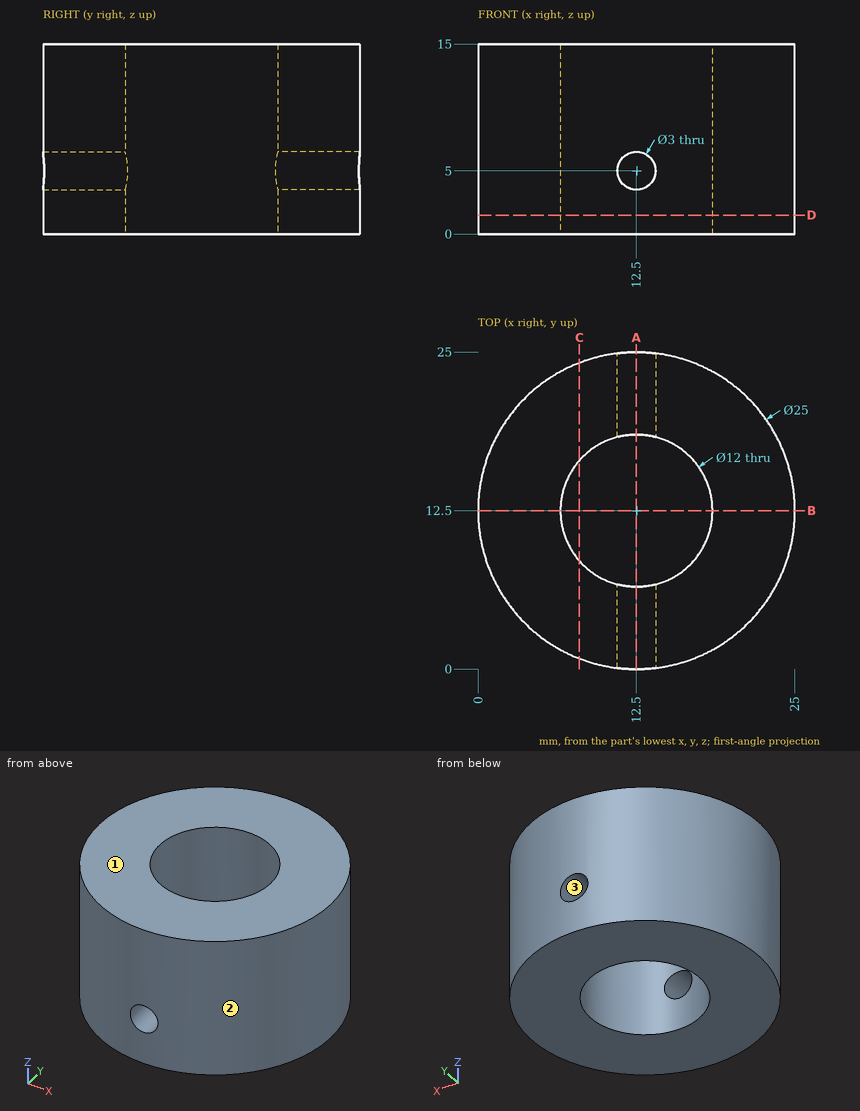
Source: three-view drawing plus pictorial views. Frame: mm from the lowest corner of the part. Round coordinates to 2 decimals unless told otherwise and drop trailing zeros. Loops run counter-clockwise (first coordinate to the right, second up) from the corner with the lowest first, then second, coordinate; pieces in that order, holes last.
1. Section query C-C on x = 8. Output: boundary loops of the cut face in (y, z), and give its area (3 significant figures).
2. Ray query, L1, parallel to Y at x = 12.5, z = 10.5; L2, parallel to Z at x = 12.5, y = 23; L3, parallel to Y at x = 14.25, z = 9.75. Return the intervals inside material, ascending.
3. Section query A-A on x = 12.5. Output: boundary loops of the cut face in (y, z), and give its area (3 significant figures).
4. Section query D-D on z = 1.5. Output: boundary loops of the cut face in (x, y).
5. Contact query for flat-ended pins moving along their axis: pin 1 (3 mm diameter, centred on x = 7.5, z = 13.5, fed in from +Y); pin 2 (14 mm diameter, centred on x = 12.5, y = 12.5, fed in from +Z); pin 3 (3 mm diameter, centred on y = 20.5, z = 11, fed in from +X); pin 4 (3 mm diameter, centred on x = 2.5, z = 9, fed in from +Y). Output: stop coordinate, or through.
6. Section query B-B on y = 12.5. Output: boundary loops of the cut face in (x, z), and give its area (3 significant figures).
7. Mould query, pull axis X, two halves, no side actions, for the marked faces 1, 2 and 3. Classes: released by +X, released by -X, zero draft, split by the parting line, or undercut.
Answers below:
1. outline: (0.84, 0) - (8.53, 0) - (8.53, 15) - (0.84, 15) - close; (16.47, 0) - (24.16, 0) - (24.16, 15) - (16.47, 15) - close
1. area: 231 mm2
2. L1: y = 0 to 6.5, 18.5 to 25
2. L2: z = 0 to 3.5, 6.5 to 15
2. L3: y = 0.12 to 6.76, 18.24 to 24.88
3. outline: (0, 0) - (6.5, 0) - (6.5, 3.5) - (0, 3.5) - close; (0, 6.5) - (6.5, 6.5) - (6.5, 15) - (0, 15) - close; (18.5, 0) - (25, 0) - (25, 3.5) - (18.5, 3.5) - close; (18.5, 6.5) - (25, 6.5) - (25, 15) - (18.5, 15) - close
3. area: 156 mm2
4. outline: circle Ø25 at (12.5, 12.5); hole circle Ø12 at (12.5, 12.5)
5. pin 1: stops at y = 24.5
5. pin 2: stops at z = 15
5. pin 3: stops at x = 23.18
5. pin 4: stops at y = 21.67
6. outline: (0, 0) - (6.5, 0) - (6.5, 15) - (0, 15) - close; (18.5, 0) - (25, 0) - (25, 15) - (18.5, 15) - close
6. area: 195 mm2
7. face 1: zero draft
7. face 2: split by the parting line
7. face 3: undercut
